Geometry: final body of the model. Coordinates: model frame, mm. A direction names the side the tool comes from. Give positions to 0.01 mm unless a question says otherwise; leave off trailing zeros. Order: outer loops, then holes, each group sorted by start corner. A loop starts at its lowest first (then second) coordinate and runs counter-clockwise, first axis right, second up. Notation, with made-up numbers: (85.5, 22) -> (102.5, 22) arc R15 ccw to (102.5, 33) -> close; hole circle Ø3 at (42, 17). An arc over 180 degrees is marked (long way). One line per question, with ' | ' between items.
from build123d import *

# Parameters (mm, degrees)
F3_R = 0.7
F4_R = 0.7


with BuildPart() as f2:
    # F2: sweep along a path in F0
    with BuildLine(Plane.XZ) as f2_path:
        Line((0, 0), (25, 0))
        ThreePointArc((25, 0), (42.6776695297, -7.3223304703), (50, -25))
        Line((50, -25), (50, -120))
    # F1 (on Right) → F2 (sweep)
    with BuildSketch(Plane.YZ):
        Polygon((-1.7320508076, 3), (-3.4641016151, 0), (-1.7320508076, -3), (1.7320508076, -3), (3.4641016151, 0), (1.7320508076, 3), align=None)
    sweep(path=f2_path.line)

    # F3
    f3_edges = [f2.edges().sort_by_distance(p)[0] for p in [
        (0, 0, 3),
        (0, -2.598076, 1.5),
        (0, -2.598076, -1.5),
        (0, 0, -3),
        (0, 2.598076, -1.5),
        (0, 2.598076, 1.5),
    ]]
    fillet(f3_edges, radius=F3_R)

    # F4
    f4_edges = [f2.edges().sort_by_distance(p)[0] for p in [
        (53, 0, -120),
        (51.5, -2.598076, -120),
        (48.5, -2.598076, -120),
        (47, 0, -120),
        (48.5, 2.598076, -120),
        (51.5, 2.598076, -120),
    ]]
    fillet(f4_edges, radius=F4_R)


solid = f2.part
1) Material intervals for probe 1 along Z at (x, y) = (15.5, 0.25); probe 2 along X at (y, z) = (-1.5, -60); probe 3 along Z at (x, y) = (29, 1.5), sorted ascending. Write a range as from..to.
Check result:
probe 1: z = -3..3 | probe 2: x = 47..53 | probe 3: z = -3.37..2.71
2) Section B-B on z = -35. Return loops of the section in (x, y), plus the area to 3 significant figures.
Check result:
outline: (47, -1.73) -> (50, -3.46) -> (53, -1.73) -> (53, 1.73) -> (50, 3.46) -> (47, 1.73) -> close | area: 31.2 mm^2
3) Section A-A on x = 7. Return loops of the section in (y, z), plus the area to 3 significant figures.
Check result:
outline: (-3.46, 0) -> (-1.73, -3) -> (1.73, -3) -> (3.46, 0) -> (1.73, 3) -> (-1.73, 3) -> close | area: 31.2 mm^2
4) Contact query for flat-ended pins moving along their axis: pin 1 Ø4 at (x, y) = (13, 0.5) entering from -Z; pin 2 Ø4 at (y, z) = (0, -15.5) entering from -X (3 decimals); pin 3 Ø4 at (y, z) = (0, -58) entering from -X. Output: stop coordinate, or through.
Check result:
pin 1: stops at z = -3 | pin 2: stops at x = 43.755 | pin 3: stops at x = 47
5) Set-up query: faces 1 (the flat face through (13, 0, -3)), 2 (the flat face through (13, -2.6, -1.5)), 3 (the flat face through (13, 2.6, 1.5)). Return all of +Z, -Z, +X, -X, +Y, -Y with unobstructed straight access to the full face (end or side cutting, diameter ignored); none if empty.
Check result:
face 1: -Z, -X, +Y, -Y | face 2: -Z, -X, -Y | face 3: +Z, +X, -X, +Y
